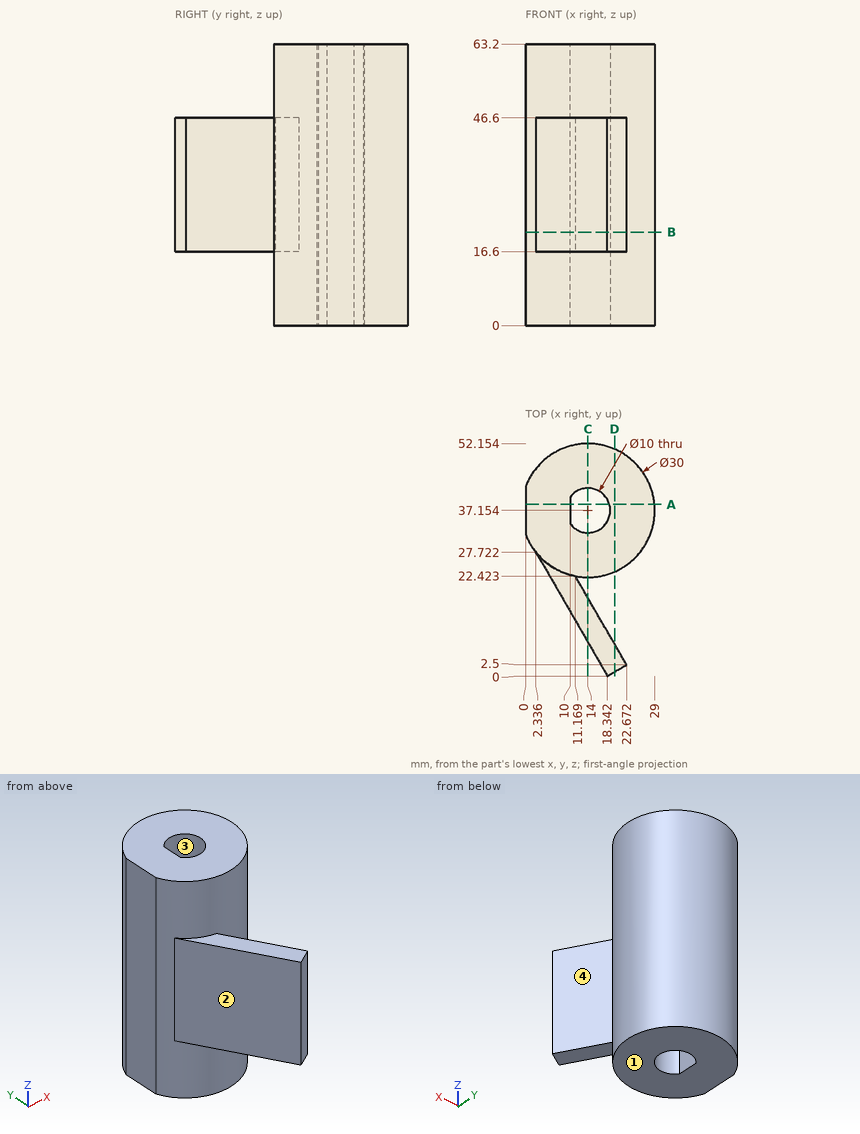
For this review, use the dimensioned drawing (mm, ordinates from the lowest corner) and the shaded views. Round coordinates to 2 decimals unless told otherwise and drop trailing zeros. Order: outer loops, then holes, each group sorted by start corner. A loop starts at its lowest first (then second) coordinate and runs counter-clockwise, first axis right, second up. Notation, with made-up numbers: (33.5, -12) - (59.5, -12) arc R23 cw to (59.5, 13) - close; hole circle Ø9 at (58, 2.5). An arc over 180 degrees is marked (long way). Use one line per item in the form item = value.
Q1. Add section D-D on x = 20. Give the boundary of the cut face in (y, z).
Response values:
outline = (0.96, 16.6) - (7.13, 16.6) - (7.13, 46.6) - (0.96, 46.6) - close; (23.41, 0) - (50.9, 0) - (50.9, 63.2) - (23.41, 63.2) - close
Q2. Mouldability with a two-part tool opening along Y and no side actions: class the marked faces 1, 2, 3 and 4 as pulls with the +Y half, pulls with the -Y half, needs draft (parallel to the pull), parting line crosses it, or undercut.
Response values:
face_1 = needs draft
face_2 = pulls with the -Y half
face_3 = undercut
face_4 = undercut
Q3. Add section A-A on y = 38.5. Give the boundary of the cut face in (x, z) (1 decimal).
Response values:
outline = (0, 0) - (10, 0) - (10, 63.2) - (0, 63.2) - close; (18.8, 0) - (28.9, 0) - (28.9, 63.2) - (18.8, 63.2) - close
Q4. Add section B-B on z = 21. Give the boundary of the cut face in (x, y).
Response values:
outline = (0, 31.77) arc R15 ccw to (2.34, 27.72) - (18.34, 0) - (22.67, 2.5) - (11.17, 22.42) arc R15 ccw (long way) to (0, 42.54) - close; hole (10, 34.15) arc R5 ccw (long way) to (10, 40.15) - close
Q5. Add section C-C on x = 14. Give the boundary of the cut face in (y, z).
Response values:
outline = (7.52, 16.6) - (17.52, 16.6) - (17.52, 46.6) - (7.52, 46.6) - close; (22.15, 0) - (32.15, 0) - (32.15, 63.2) - (22.15, 63.2) - close; (42.15, 0) - (52.15, 0) - (52.15, 63.2) - (42.15, 63.2) - close
Q6. Clearance check with flat-ended pins moving along their axes: P1, Ø10, axis at y = 20, z = 25, coming from the -X side; P2, Ø6, axis at x = 25.5, z = 48.5, coming from the +Y side; P3, Ø1.5, axis at x = 8.5, z = 47, coming from the +Y side. State where each tip first meets the part, or that it passes through.
Response values:
P1 = 3.91
P2 = 49.51
P3 = 51.38
Q7. To check wall thickness, follow line 1 (Y direction, x = 13.5, z = 31) (1 decimal); line 2 (Y direction, x = 15.25, z = 37) (1 decimal); line 3 (X direction, y = 37.5, z = 40). State the ranges of each line that lie inside material, in increasing order.
Response values:
line_1 = 8.4 to 18.4, 22.2 to 32.2, 42.1 to 52.1
line_2 = 5.4 to 15.4, 22.2 to 32.3, 42 to 52.1
line_3 = 0 to 10, 18.99 to 29
